Solid Edge part; units mm, degrees
sketch "Sketch1" plane through (0, 0, 0) normal (0, 0, 1) x (1, 0, 0)
  line L0 (-67.5, -67.5) -> (67.5, -67.5)
  line L1 (67.5, -67.5) -> (67.5, 67.5)
  line L2 (67.5, 67.5) -> (32, 67.5)
  line L3 (32, 131.5) -> (32, 67.5)
  line L4 (-32, 131.5) -> (32, 131.5)
  line L5 (-32, 67.5) -> (-32, 131.5)
  line L6 (-32, 67.5) -> (-67.5, 67.5)
  line L7 (-67.5, 67.5) -> (-67.5, -67.5)
extrude "Protrusion1" add sketch "Sketch1" along normal mid plane 1
sketch "Sketch2" plane through (0, 32, -0.5) normal (0, 0, -1) x (-1, 0, 0)
  line L0 (11, -39.5) -> (12, -39.5)
  line L1 (12, -39.5) -> (12, -24.5)
  line L2 (12, -24.5) -> (11, -24.5)
  line L3 (11, -24.5) -> (11, -39.5)
  line L4 (52, -39.5) -> (53, -39.5)
  line L5 (53, -39.5) -> (53, -24.5)
  line L6 (53, -24.5) -> (52, -24.5)
  line L7 (52, -24.5) -> (52, -39.5)
  line L8 (-11, -39.5) -> (-12, -39.5)
  line L9 (-12, -39.5) -> (-12, -24.5)
  line L10 (-12, -24.5) -> (-11, -24.5)
  line L11 (-11, -24.5) -> (-11, -39.5)
  line L12 (-52, -39.5) -> (-53, -39.5)
  line L13 (-53, -39.5) -> (-53, -24.5)
  line L14 (-53, -24.5) -> (-52, -24.5)
  line L15 (-52, -24.5) -> (-52, -39.5)
  dimension "D1" = 11
  dimension "D2" = 11
extrude "Wyciągnięcie_9" add sketch "Sketch2" along normal blind 28
sketch "Sketch3" plane through (-53, 0, -14.5) normal (-1, 0, 0) x (0, 1, 0)
  circle A0 centre (0, 6.5) radius 2.5
extrude "Cutout1" cut sketch "Sketch3" against normal through all
sketch "Sketch4" plane through (0, 32, -0.5) normal (0, 0, -1) x (0, 1, 0)
  line L0 (-81, 27) -> (-66, 27)
  line L1 (-66, 27) -> (-66, 28)
  line L2 (-66, 28) -> (-81, 28)
  line L3 (-81, 28) -> (-81, 27)
  line L4 (-81, -28) -> (-66, -28)
  line L5 (-66, -28) -> (-66, -27)
  line L6 (-66, -27) -> (-81, -27)
  line L7 (-81, -27) -> (-81, -28)
  dimension "D1" = 66
  dimension "D2" = 81
  dimension "D3" = 81
  dimension "D4" = 66
  dimension "D5" = 0.0001
extrude "Wyciągnięcie_10" add sketch "Sketch4" along normal blind 24
sketch "Sketch5" plane through (28, -41.5, -12.5) normal (1, 0, 0) x (0, 1, 0)
  circle A0 centre (0, -3) radius 2.5
extrude "Cutout2" cut sketch "Sketch5" against normal up to next
sketch "Sketch6" plane through (-27, -41.5, -12.5) normal (1, 0, 0) x (0, 1, 0)
  circle A0 centre (0, -3) radius 2.5
extrude "Cutout3" cut sketch "Sketch6" against normal up to next
sketch "Sketch7" plane through (0, 32, 0.5) normal (0, 0, 1) x (1, 0, 0)
  line L0 (0.25, 67.25) -> (31.5, 67.25)
  line L1 (31.5, 67.25) -> (31.5, 67.75)
  line L2 (31.5, 67.75) -> (0.25, 67.75)
  line L3 (0.25, 67.75) -> (0.25, 99)
  line L4 (0.25, 99) -> (-0.25, 99)
  line L5 (-0.25, 99) -> (-0.25, 67.75)
  line L6 (-0.25, 67.75) -> (-31.5, 67.75)
  line L7 (-31.5, 67.75) -> (-31.5, 67.25)
  line L8 (-31.5, 67.25) -> (-0.25, 67.25)
  line L9 (-0.25, 67.25) -> (-0.25, 36)
  line L10 (-0.25, 36) -> (0.25, 36)
  line L11 (0.25, 36) -> (0.25, 67.25)
extrude "Wyciągnięcie_11" add sketch "Sketch7" along normal blind 46
sketch "Sketch8" plane through (0, 32, 0.5) normal (0, 0, 1) x (1, 0, 0)
  circle A0 centre (5.25, 62.25) radius 2
  circle A1 centre (-5.25, 62.25) radius 2
  circle A2 centre (-5.25, 72.75) radius 2
  circle A3 centre (5.25, 72.75) radius 2
  dimension "D1" = 5.25
  dimension "D2" = 5.25
  dimension "D3" = 5.25
  dimension "D4" = 5.25
extrude "Cutout4" cut sketch "Sketch8" against normal up to next
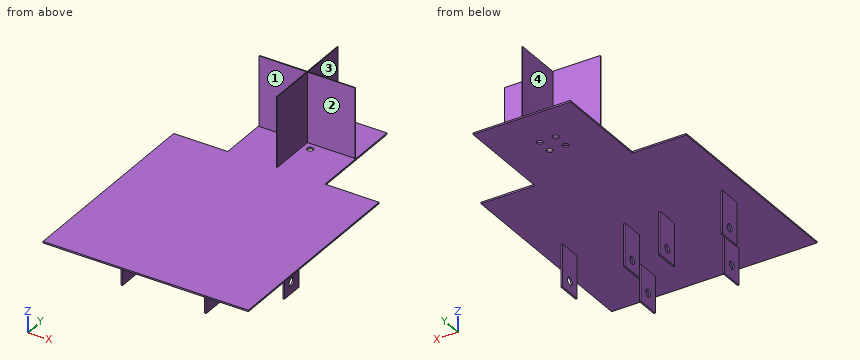
Part model, mm, in its own coordinate system. Face numbers are marked on the shaded views. A direction names the side the tool comes from. Round coordinates to 2 decimals unless told otherwise and drop trailing zeros. Write each loop counter-clockwise with the first axis right and the second up, starting at its lowest first coordinate (ties: lowest second). Pieces come first, ordered by that corner, then holes.
Item 1: Which spindle directions (+Z, -Z, +X, -X, +Y, -Y) get a long thin tool onto all of the face, cutting with end or side? Do the marked faces 1, 2, 3 and 4. Say none if no direction does.
Results:
face 1: +Z, -X, -Y
face 2: +Z, +X, -Y
face 3: +Z, +X, +Y
face 4: +Z, -X, +Y
Item 2: Cut at C-C, the plane x = 48. Give the cut face in (y, z), plus the area to 3 significant figures.
Results:
outline: (-67.5, -0.5) - (67.5, -0.5) - (67.5, 0.5) - (-67.5, 0.5) - close
area: 135 mm2
Item 3: Cut at B-B, the plane z = 25. Give the cut face in (x, y).
Results:
outline: (-31.5, 99.25) - (-0.25, 99.25) - (-0.25, 68) - (0.25, 68) - (0.25, 99.25) - (31.5, 99.25) - (31.5, 99.75) - (0.25, 99.75) - (0.25, 131) - (-0.25, 131) - (-0.25, 99.75) - (-31.5, 99.75) - close
Item 4: Drop flat-ended pins along their axis: pin 1 Ø1.5 at (x, z) = (-22, 8.5) entering from +Y; pin 2 Ø0.6 at (y, z) = (99.5, 16.5) entering from -X; pin 3 Ø6 at (y, z) = (0, -21) entering from +X; pin 4 Ø5 at (x, z) = (34, 0.5) entering from +Y. Give the stop position or say it passes through.
Results:
pin 1: stops at y = 99.75
pin 2: stops at x = -31.5
pin 3: stops at x = 53
pin 4: stops at y = 131.5
Item 5: Cut at A-A, the plane y = -41.5. Give the cut face in (x, z).
Results:
outline: (-67.5, -0.5) - (-28, -0.5) - (-28, -13) - (-27, -13) - (-27, -0.5) - (27, -0.5) - (27, -13) - (28, -13) - (28, -0.5) - (67.5, -0.5) - (67.5, 0.5) - (-67.5, 0.5) - close; (-28, -24.5) - (-27, -24.5) - (-27, -18) - (-28, -18) - close; (27, -24.5) - (28, -24.5) - (28, -18) - (27, -18) - close
Item 6: Cut at D-D, the plane z = -21. Count the separate pieces of the cut face and the enclosed holes in it, plus the area to 3 significant figures.
Results:
separate pieces: 10
enclosed holes: 0
area: 70.0 mm2
Item 7: Probe L1, parallel to X at y = 0.5, z = -3; L2, parallel to Y at x = 5.25, z = 0.15; L3, parallel to Y at x = 11.4, z = -21. List the from-to ranges inside material, lowest first.
Results:
L1: x = -53 to -52, -12 to -11, 11 to 12, 52 to 53
L2: y = -67.5 to 92.25, 96.25 to 102.75, 106.75 to 131.5
L3: y = -7.5 to -2.5, 2.5 to 7.5
